from build123d import *

# Parameters (mm, degrees)
SKETCH1_W           = 20
SKETCH1_H           = 13.7
SKETCH1_R           = 0.405
BOSS_EXTRUDE1_DEPTH = 1.16
CHAMFER1_SIZE       = 0.5


with BuildPart() as part:
    # Sketch1 → Boss-Extrude1 (new body)
    with BuildSketch(Plane(origin=(0, 0, 0), x_dir=(1, 0, 0), z_dir=(0, 1, 0))):
        Rectangle(SKETCH1_W, SKETCH1_H)
        with Locations(Location((-8, -5.08, 0), (0, 0, 270))):
            Circle(SKETCH1_R, mode=Mode.SUBTRACT)
        with Locations(Location((-8, -2.54, 0), (0, 0, 270))):
            Circle(SKETCH1_R, mode=Mode.SUBTRACT)
        with Locations(Location((-8, 0, 0), (0, 0, 270))):
            Circle(SKETCH1_R, mode=Mode.SUBTRACT)
        with Locations(Location((-8, 2.54, 0), (0, 0, 270))):
            Circle(SKETCH1_R, mode=Mode.SUBTRACT)
        with Locations(Location((-8, 5.08, 0), (0, 0, 270))):
            Circle(SKETCH1_R, mode=Mode.SUBTRACT)
    extrude(amount=BOSS_EXTRUDE1_DEPTH)

    # Chamfer1
    chamfer1_edges = [part.edges().sort_by_distance(p)[0] for p in [
        (-10, 0.58, -6.85),
        (10, 0.58, -6.85),
        (10, 0.58, 6.85),
        (-10, 0.58, 6.85),
    ]]
    chamfer(chamfer1_edges, length=CHAMFER1_SIZE)


solid = part.part
Here's how the part is built. I have some questions about the finished solid (model axes, mm). Round coordinates to 2 decimals unless told otherwise and drop trailing zeros. Write each loop counter-clockwise with the first axis right and the second up, starting at its lowest first coordinate (ties: lowest second). Pieces come first, ordered by that corner, then holes.
1. Suppose I cut it at A-A (x = -8). List the corners of the cut face in (y, z) for me (3 decimals).
2. If we mould it in two halves opening along X, with no side actions, what happens to faces 1 (the flat face through (0, 1, 6.85)), 2 (the cylindrical face through (-7.66, 0.57, 2.76)), 3 (the flat face through (-10, 1, 0)), 4 (the cylindrical face through (-7.6, 0.57, -0.05))? For each: released by +X, released by -X, zero draft, split by the parting line, or undercut.
3. I need wall thicknesses on L1, parallel to X at y = 1.05, z = -2.5; L2, parallel to X at y = 0.9, z = -0.25. Which ranges of each line are inside material? Lowest first, please.
4. Suppose I cut it at C-C (z = 5). List the corners of the cut face in (x, y) for me, and give its area (3 significant figures).
5. Suppose I cut it at B-B (z = 2.54). List the corners of the cut face in (x, y) for me (3 decimals), and give its area (3 significant figures).
Answer sheet:
1. outline: (0, -6.85) - (1.16, -6.85) - (1.16, -5.485) - (0, -5.485) - close; (0, -4.675) - (1.16, -4.675) - (1.16, -2.945) - (0, -2.945) - close; (0, -2.135) - (1.16, -2.135) - (1.16, -0.405) - (0, -0.405) - close; (0, 0.405) - (1.16, 0.405) - (1.16, 2.135) - (0, 2.135) - close; (0, 2.945) - (1.16, 2.945) - (1.16, 4.675) - (0, 4.675) - close; (0, 5.485) - (1.16, 5.485) - (1.16, 6.85) - (0, 6.85) - close
2. face 1: zero draft
2. face 2: undercut
2. face 3: released by -X
2. face 4: undercut
3. L1: x = -10 to -8.4, -7.6 to 10
3. L2: x = -10 to -8.32, -7.68 to 10
4. outline: (-10, 0) - (-8.4, 0) - (-8.4, 1.16) - (-10, 1.16) - close; (-7.6, 0) - (10, 0) - (10, 1.16) - (-7.6, 1.16) - close
4. area: 22.3 mm2
5. outline: (-10, 0) - (-8.405, 0) - (-8.405, 1.16) - (-10, 1.16) - close; (-7.595, 0) - (10, 0) - (10, 1.16) - (-7.595, 1.16) - close
5. area: 22.3 mm2
